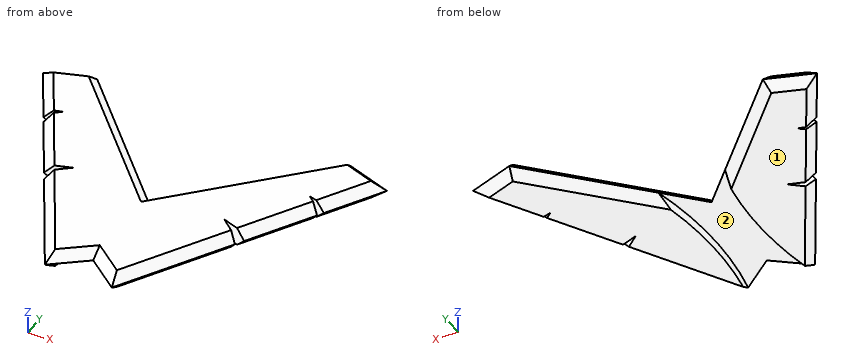
```python
from build123d import *

# Parameters (mm, degrees)
F1_DEPTH = 6.35
F3_DEPTH = 3.175
F4_SIZE  = 3.17499


# Not quite as in the source:
# - a fillet or chamfer is up to 0.001 mm smaller than in the source, because OpenCascade refuses the exact size


with BuildPart() as f1:
    # F0 (on Top) → F1 (new body)
    with BuildSketch(Plane.XY):
        Polygon((-21.1028610796, 36.5512275749), (-11.7370359251, 20.3291425525), (0, 29.516665265), (11.7370359251, 20.3291425525), (33.4666037048, 57.9658579735), (26.5181194991, 63.6764243245), (35.1014384706, 60.7974748498), (47.9729409095, 83.0915710438), (43.2239025831, 86.8056491017), (49.1863254635, 85.1932147405), (60.325, 104.4859649666), (44.45, 109.9852262806), (0, 63.5), (-44.45, 109.9852262806), (-60.325, 104.4859649666), (-49.1863254635, 85.1932147405), (-43.2239025831, 86.8056491017), (-47.9729409095, 83.0915710438), (-35.1014384706, 60.7974748498), (-26.5181194991, 63.6764243245), (-33.4666037048, 57.9658579735), align=None)
    extrude(amount=F1_DEPTH)

    # F2 (on face) → F3 (cut)
    with BuildSketch(Plane(origin=(0, 0, 0), x_dir=(1, 0, 0), z_dir=(0, 0, -1))):
        with BuildLine():
            ThreePointArc((11.7370359251, -75.7744380392), (8.6743378245, -48.0517902958), (11.7370359251, -20.3291425525))
            Line((11.7370359251, -20.3291425525), (0, -29.516665265))
            Line((0, -29.516665265), (-11.7370359251, -20.3291425525))
            ThreePointArc((-11.7370359251, -20.3291425525), (-8.6743378245, -48.0517902958), (-11.7370359251, -75.7744380392))
            Line((-11.7370359251, -75.7744380392), (0, -63.5))
            Line((0, -63.5), (11.7370359251, -75.7744380392))
        make_face()
        Polygon((-11.7370359251, -75.7744380392), (11.7370359251, -75.7744380392), (0, -63.5), align=None)
        Polygon((0, -29.516665265), (11.7370359251, -20.3291425525), (-11.7370359251, -20.3291425525), align=None)
    extrude(amount=-F3_DEPTH, mode=Mode.SUBTRACT)

    # F4 (size 3.175 in the source; OpenCascade refuses exactly that, so slightly less here)
    f4_edges = [f1.edges().sort_by_distance(p)[0] for p in [
        (22.60182, 39.1475, 6.35),
        (22.60182, 39.1475, 0),
        (41.53719, 71.944523, 6.35),
        (41.53719, 71.944523, 0),
        (54.755663, 94.83959, 6.35),
        (54.755663, 94.83959, 0),
        (52.3875, 107.235596, 6.35),
        (52.3875, 107.235596, 0),
        (22.225, 86.742613, 6.35),
        (28.093518, 92.879832, 0),
        (5.868518, 24.922904, 6.35),
        (-5.868518, 24.922904, 6.35),
        (-22.225, 86.742613, 6.35),
        (-28.093518, 92.879832, 0),
        (-52.3875, 107.235596, 6.35),
        (-52.3875, 107.235596, 0),
        (-54.755663, 94.83959, 6.35),
        (-54.755663, 94.83959, 0),
        (-41.53719, 71.944523, 6.35),
        (-41.53719, 71.944523, 0),
        (-22.60182, 39.1475, 6.35),
        (-22.60182, 39.1475, 0),
    ]]
    chamfer(f4_edges, length=F4_SIZE)


solid = f1.part
```
Check sheet for the modelled part. Datum: model origin and axes. Units: mm. Face numbers are marked on the shaded views. Give positions to 0.01 mm unless a question says otherwise; leave off trailing zeros. Order: outer loops, then holes, each group sorted by start corner. A loop starts at its lowest first (then second) coordinate and runs counter-clockwise, first axis right, second up. Notation, with made-up numbers: M 82,3 L 122,3 A10 cw 122,13 Z; hole C 70,61.5 d6. An arc over 180 degrees is marked long. Answer in a Markdown table with one row per item.
1) Gauge pin test, flat ends, axial feed: P1, Ø7, axis at x = -1.5, y = 36, coming from the -Z side (3 decimals); P2, Ø2, axis at y = 39, z = 2, coming from the +X side. Record the tip position at first contact, or that the pin passes through.
Filled sheet:
| item | result |
|---|---|
| P1 | stops at z = 3.175 |
| P2 | stops at x = 22.45 |
2) Cross-section at A-A, the plane z = 1. Enter the section's corners in (x, y), plus the area to 3 significant figures.
Filled sheet:
| item | result |
|---|---|
| outline | M -57.12,103.29 L -47.01,85.78 L -43.22,86.81 L -46.24,84.44 L -33,61.5 L -26.52,63.68 L -31.76,59.37 L -11.07,23.52 A127 ccw -10.91,71.76 L -45.06,107.47 Z; M 10.91,71.76 A127 ccw 11.07,23.52 L 31.76,59.37 L 26.52,63.68 L 33,61.5 L 46.24,84.44 L 43.22,86.81 L 47.01,85.78 L 57.12,103.29 L 45.06,107.47 Z |
| area | 2,930 mm2 |
3) Release check for a two-part mould opening along X. For the marked faces 1 and 2 record: +X half, -X half, draft (parallel to the pull), parting line (faces both ways), or undercut.
Filled sheet:
| item | result |
|---|---|
| face 1 | draft |
| face 2 | undercut |
4) Thickness scan on L1, parallel to X at y = 54.5, z = 2.5; L2, parallel to X at y = 72.5, z = 3.5; L3, parallel to Y at x = 44, z = 1.25. Record the ranges inside material, lowest first. Write a range as [from, to].
Filled sheet:
| item | result |
|---|---|
| L1 | x = [-30.69, -8.84], [8.84, 30.69] |
| L2 | x = [-41.48, -9.06], [9.06, 41.48] |
| L3 | y = [80.06, 86.2], [86.6, 106.73] |
